Model file for the job. Use its own axes, mm. A direction names the side the tool comes from. Give positions to 0.01 mm unless a question says otherwise; leave off trailing zeros. Order: outer loops, then holes, each group sorted by start corner. A loop starts at its lowest first (then second) coordinate and runs counter-clockwise, first axis right, second up. Notation, with made-up numbers: (78, 57) - (128, 57) arc R17 ccw to (128, 88) - close; hole circle Ø10 at (43, -31). An arc over 180 degrees is marked (long way). Use CSV: the item, a comma, the result in double quotes. Start each with the question number.
(1) Pull direction Y, two halves, no side cores. Call faces 3 (the conical face through (36.96, -11.64, 54.69)), 4 (the conical face through (6.155, -1.938, 26.344)), 5 (the flat face through (6, 19, 75)), 6 (the conical face through (-1.349, 6.077, 26.549)): +Y half, -Y half, draft (parallel to the pull), parting line (faces both ways), or undercut.
(2) Probe L1, parallel to Y at x = -8, z = 63; L2, parallel to X at y = 13, z = 71.5; L3, parallel to Y at x = -1, z = 46.5. List the from-to ranges inside material, lowest first.
(3) Drop flat-ended pins along their axis: pin 1 Ø8 at (x, y) = (-41.5, -27) entering from +Z; pin 2 Ø6 at (y, z) = (27.5, 47.5) entering from +X; pin 3 Ø10 at (y, z) = (-27, 54) entering from -X; pin 4 Ø12 at (y, z) = (-41.5, 66) entering from +X. Give the stop position or say it passes through.
(4) Band-saw the part on A-A, the plane z = 63.5. Give the cut face in (x, y).
(5) Band-saw the part on B-B, the plane z = 50.5. Give the cut face in (x, y), then the cut area to 3 significant figures.
(6) Tool access for faces 1 (the flat face through (4, 16, 43.4)), 2 (the conical face through (-3.94, 17.744, 59.971)): list every direction of +Z, -Z, +X, -X, +Y, -Y with a clear straight run to the whole face (end or side of a thin tool).
from build123d import *


# Not quite as in the source:
# - a fillet or chamfer that OpenCascade refuses, or shapes differently, is made with other operations: its cross-section is extruded or revolved along the edge and cut away or added


with BuildPart() as f1:
    # F0 (on Front) → F1 (revolve)
    with BuildSketch(Plane.XZ):
        Polygon((64.667229809, 0), (65, 0), (29, 75), (19, 75), (17.3, 44), (16.3, 44), (0, 15.7675718366), (0, 15.1675718366), (16.3, 43.4), (17.8679982822, 43.4), (19.5679982822, 74.4), (28.955229809, 74.4), align=None)
    revolve(axis=Axis((0, 0, 43.4963169246), (0, 0, -1)))

    # F2: fillet of radius 1.5 on 1 edges, made by hand

    # F2_s1 → F2_t2 (revolve)
    with BuildSketch(Plane.XZ):
        with BuildLine():
            ThreePointArc((17.3744099359, 45.3568870669), (17.0526414639, 44.5078566678), (16.3, 44))
            Line((16.3, 44), (16.3084667935, 43.9712195655))
            ThreePointArc((16.3084667935, 43.9712195655), (16.8, 43.97), (17.3, 43.97))
            Line((17.3, 43.97), (17.3299549922, 43.9983573069))
            Line((17.3299549922, 43.9983573069), (17.4043649282, 45.3552443738))
            Line((17.4043649282, 45.3552443738), (17.3744099359, 45.3568870669))
        make_face()
    revolve(axis=Axis((0, 0, 44), (0, 0, -1)))


solid = f1.part
Answer block:
1,face 3,"parting line"
1,face 4,"undercut"
1,face 5,"draft"
1,face 6,"undercut"
2,L1,"y = -33.83 to -33.48, -17.17 to -16.51, 16.51 to 17.17, 33.48 to 33.83"
2,L2,"x = -27.79 to -27.42, -14.41 to -13.59, 13.59 to 14.41, 27.42 to 27.79"
2,L3,"y = -42.67 to -42.34, -18.01 to -17.41, 17.41 to 18.01, 42.34 to 42.67"
3,pin 1,"stops at z = 40.6"
3,pin 2,"stops at x = 35"
3,pin 3,"stops at x = -33.37"
3,pin 4,"passes through"
4,outline,"circle Ø69.04 at (0, 0); circle Ø37.94 at (0, 0); hole circle Ø68.37 at (0, 0); hole circle Ø36.74 at (0, 0)"
5,outline,"circle Ø81.52 at (0, 0); circle Ø36.51 at (0, 0); hole circle Ø80.85 at (0, 0); hole circle Ø35.31 at (0, 0)"
5,area,"153 mm2"
6,face 1,"-Z"
6,face 2,"+Z"
